Verification items for the finished model (mm, model axes). Face numbers are marked on the shaded views. Give positions to 0.01 mm unless a question says otherwise; leave off trailing zeros. Write item = value, one per line.
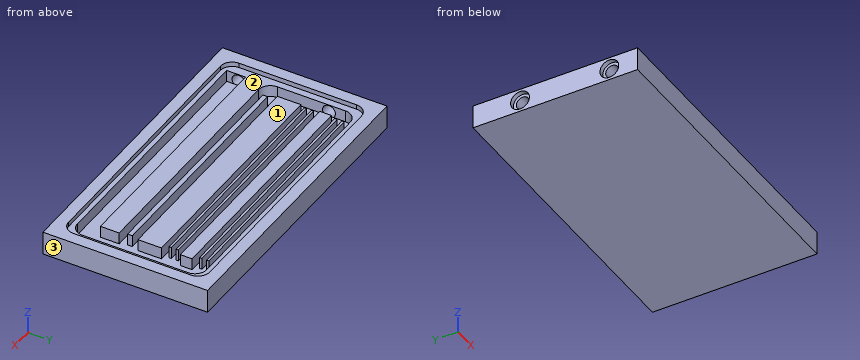
from build123d import *

# Parameters (mm, degrees)
ESQUISSE1_W                                 = 130
ESQUISSE1_H                                 = 70
BOSS_EXTRU_1_DEPTH                          = 10
ENL_V_MAT_EXTRU_1_DEPTH                     = 2
ESQUISSE20_W                                = 101.033933646
ESQUISSE20_H                                = 5
ESQUISSE20_H_2                              = 10
ENL_V_MAT_EXTRU_3_DEPTH                     = 5
CHAMBRAGE_POUR_VIS_SIX_PANS_CREUX_2_R       = 2.75
CHAMBRAGE_POUR_VIS_SIX_PANS_CREUX_M52_DEPTH = 7.966066354
CHAMBRAGE_POUR_VIS_SIX_PANS_CREUX_3_OU_R    = 4
CHAMBRAGE_POUR_VIS_SIX_PANS_CREUX_3_OU_R_2  = 2.75
CHAMBRAGE_POUR_VIS_SIX_PANS_CREUX_3_DEPTH   = 2
CHAMBRAGE_START                             = 7.966066354
CHAMBRAGE_POUR_VIS_SIX_PANS_CREUX_4_OU_R    = 2.75
CHAMBRAGE_POUR_VIS_SIX_PANS_CREUX_4_DEPTH   = 0.858319246
ESQUISSE23_W                                = 98
ESQUISSE23_H                                = 1
ESQUISSE23_H_2                              = 2
BOSS_EXTRU_2_DEPTH                          = 5


# Read off the part's stored shape, not the designer's step: Chambrage pour vis à six pans creux M52
with BuildPart() as part:
    # Esquisse1 → Boss.-Extru.1 (new body)
    with BuildSketch(Plane.XY):
        with Locations((65, 35)):
            Rectangle(ESQUISSE1_W, ESQUISSE1_H)
    extrude(amount=BOSS_EXTRU_1_DEPTH)

    # Esquisse18 → Enlèv. mat.-Extru.1 (cut)
    with BuildSketch(Plane.XY.offset(10)):
        with BuildLine():
            Line((10, 5), (120, 5))
            ThreePointArc((120, 5), (123.535533906, 6.464466094), (125, 10))
            Line((125, 10), (125, 60))
            ThreePointArc((125, 60), (123.535533906, 63.535533906), (120, 65))
            Line((120, 65), (10, 65))
            ThreePointArc((10, 65), (6.464466094, 63.535533906), (5, 60))
            Line((5, 60), (5, 10))
            ThreePointArc((5, 10), (6.464466094, 6.464466094), (10, 5))
        make_face()
    extrude(amount=-ENL_V_MAT_EXTRU_1_DEPTH, mode=Mode.SUBTRACT)

    # Esquisse20 → Enlèv. mat.-Extru.3 (cut)
    with BuildSketch(Plane.XY.offset(8)):
        with BuildLine():
            Line((12.966066354, 62), (117, 62))
            ThreePointArc((117, 62), (120.535533906, 60.535533906), (122, 57))
            Line((122, 57), (122, 12))
            ThreePointArc((122, 12), (120.535533906, 8.464466094), (117, 7))
            Line((117, 7), (8.8243856, 7))
            Line((8.8243856, 7), (8.8243856, 15))
            Line((8.8243856, 15), (114, 15))
            Line((114, 15), (114, 23))
            Line((114, 23), (12.966066354, 23))
            ThreePointArc((12.966066354, 23), (9.430532448, 24.464466094), (7.966066354, 28))
            Line((7.966066354, 28), (7.966066354, 57))
            ThreePointArc((7.966066354, 57), (9.430532448, 60.535533906), (12.966066354, 62))
        make_face()
        with Locations((63.483033177, 51.5)):
            Rectangle(ESQUISSE20_W, ESQUISSE20_H, mode=Mode.SUBTRACT)
        with Locations((63.483033177, 36)):
            Rectangle(ESQUISSE20_W, ESQUISSE20_H_2, mode=Mode.SUBTRACT)
    extrude(amount=-ENL_V_MAT_EXTRU_3_DEPTH, mode=Mode.SUBTRACT)

    # Chambrage pour vis _ six pans creux  2 → Chambrage pour vis à six pans creux M52 (cut)
    with BuildSketch(Plane.YZ):
        with Locations((12, 5)):
            Circle(CHAMBRAGE_POUR_VIS_SIX_PANS_CREUX_2_R)
        with Locations((50, 5)):
            Circle(CHAMBRAGE_POUR_VIS_SIX_PANS_CREUX_2_R)
    extrude(amount=CHAMBRAGE_POUR_VIS_SIX_PANS_CREUX_M52_DEPTH, mode=Mode.SUBTRACT)

    # Chambrage pour vis _ six pans creux 3 ou → Chambrage pour vis _ six pans creux  3 (cut)
    # profile 1 of 2: a face of its own
    with BuildSketch(Plane.YZ):
        with Locations((12, 5)):
            Circle(CHAMBRAGE_POUR_VIS_SIX_PANS_CREUX_3_OU_R)
        with Locations((12, 5)):
            Circle(CHAMBRAGE_POUR_VIS_SIX_PANS_CREUX_3_OU_R_2, mode=Mode.SUBTRACT)
    # profile 2 of 2: a face of its own
    with BuildSketch(Plane.YZ):
        with Locations((50, 5)):
            Circle(CHAMBRAGE_POUR_VIS_SIX_PANS_CREUX_3_OU_R)
        with Locations((50, 5)):
            Circle(CHAMBRAGE_POUR_VIS_SIX_PANS_CREUX_3_OU_R_2, mode=Mode.SUBTRACT)
    extrude(amount=CHAMBRAGE_POUR_VIS_SIX_PANS_CREUX_3_DEPTH, mode=Mode.SUBTRACT)

    # Chambrage pour vis _ six pans creux 4 ou → Chambrage pour vis _ six pans creux  4 (cut)
    with BuildSketch(Plane.YZ.offset(CHAMBRAGE_START)):
        with Locations((12, 5)):
            Circle(CHAMBRAGE_POUR_VIS_SIX_PANS_CREUX_4_OU_R)
    extrude(amount=CHAMBRAGE_POUR_VIS_SIX_PANS_CREUX_4_DEPTH, mode=Mode.SUBTRACT)

    # Esquisse23 → Boss.-Extru.2 (add)
    with BuildSketch(Plane.XY.offset(3)):
        with Locations((62.966066354, 59.5)):
            Rectangle(ESQUISSE23_W, ESQUISSE23_H)
        with Locations((62.966066354, 56.5)):
            Rectangle(ESQUISSE23_W, ESQUISSE23_H)
        with Locations((62.966066354, 46.5)):
            Rectangle(ESQUISSE23_W, ESQUISSE23_H)
        with Locations((62.966066354, 43.5)):
            Rectangle(ESQUISSE23_W, ESQUISSE23_H)
        with Locations((63.966066354, 27)):
            Rectangle(ESQUISSE23_W, ESQUISSE23_H_2)
    extrude(amount=BOSS_EXTRU_2_DEPTH)


solid = part.part
1) Depth check by flat-ended pin: P1, Ø0.6, axis at x = 65.5, y = 27, coming from the +Z side. Enter the tip coordinate at first touch or a pass-through.
From the geometry:
P1 = 8
2) Draft check along Y on the marked faces 1, 2 and 3. Enter one of: +Y half, -Y half, draft (parallel to the pull), parting line (faces both ways), or undercut.
From the geometry:
face_1 = undercut
face_2 = undercut
face_3 = draft
3) Material ranges on probe 1 along Y at (x, z) = (6.4, 5); probe 2 along X at (y, z) = (43.5, 4); probe 3 along X at (y, z) = (35, 7.75), recorded low to high. Write a range as from..to.
From the geometry:
probe_1 = 0..9.25, 14.75..47.25, 52.75..70
probe_2 = 0..7.97, 13.97..111.97, 122..130
probe_3 = 0..7.97, 12.97..114, 122..130
4) Cross-section at A-A on z = 5. Count the separate pieces of the cut face and the enclosed holes in it, plus the area to 3 significant figures.
From the geometry:
separate_pieces = 9
enclosed_holes = 0
area = 5,710 mm^2
